Geometry: final body of the model. Coordinates: model frame, mm. A direction names the side the tool comes from. Round coordinates to 2 decimals unless told otherwise and drop trailing zeros. Answer as a JSON object with one key per item and string values.
from build123d import *

# Parameters (mm, degrees)
SKETCH1_R           = 100
BOSS_EXTRUDE1_DEPTH = 50
CUT_EXTRUDE1_DEPTH  = 151
CIRPATTERN1_COUNT   = 6
FILLET1_R           = 3
SKETCH3_R           = 3
CUT_EXTRUDE2_DEPTH  = 151.000000067


with BuildPart() as part:
    # Sketch1 → Boss-Extrude1 (new body)
    with BuildSketch(Plane.XY):
        Circle(SKETCH1_R)
    extrude(amount=BOSS_EXTRUDE1_DEPTH)

    # Sketch2 → Cut-Extrude1 (cut, through all)
    with BuildSketch(Plane.XY.offset(50)):
        with BuildLine():
            Line((0, 90), (0, 10))
            ThreePointArc((0, 10), (2.588190451, 9.659258263), (5, 8.660254038))
            Line((5, 8.660254038), (45, 77.942286341))
            ThreePointArc((45, 77.942286341), (23.293714059, 86.933324366), (0, 90))
        make_face()
    cut_extrude1 = extrude(amount=-CUT_EXTRUDE1_DEPTH, mode=Mode.SUBTRACT)

    # CirPattern1: Cut-Extrude1 ×6 about axis
    cirpattern1_axis = Axis((0, 0, 0), (0, 0, 1))
    for i in range(1, CIRPATTERN1_COUNT):
        add(cut_extrude1.rotate(cirpattern1_axis, i * 360 / CIRPATTERN1_COUNT), mode=Mode.SUBTRACT)

    # Fillet1
    fillet1_edges = [part.edges().sort_by_distance(p)[0] for p in [
        (45, 77.942286341, 25),
        (5, 8.660254038, 25),
        (0, 10, 25),
        (0, 90, 25),
        (-100, 0, 0),
        (90, 0, 25),
        (10, 0, 25),
        (8.660254038, 5, 25),
        (77.942286341, 45, 25),
        (45, -77.942286341, 25),
        (5, -8.660254038, 25),
        (8.660254038, -5, 25),
        (-100, 0, 50),
        (77.942286341, -45, 25),
        (-90, 0, 25),
        (-10, 0, 25),
        (-8.660254038, -5, 25),
        (-77.942286341, -45, 25),
        (-45, -77.942286341, 25),
        (-5, -8.660254038, 25),
        (0, -10, 25),
        (0, -90, 25),
        (-45, 77.942286341, 25),
        (-5, 8.660254038, 25),
        (-8.660254038, 5, 25),
        (-77.942286341, 45, 25),
    ]]
    fillet(fillet1_edges, radius=FILLET1_R)

    # Sketch3 → Cut-Extrude2 (cut, through all)
    with BuildSketch(Plane.XY.offset(50)):
        Circle(SKETCH3_R)
    extrude(amount=-CUT_EXTRUDE2_DEPTH, mode=Mode.SUBTRACT)


solid = part.part
1) Section query A-A (y = -27). Count the separate pieces of the cut face and the enclosed holes in it, and give its area (3 significant figures).
Results:
{"separate pieces": "4", "enclosed holes": "0", "area": "5,330 mm2"}
2) Reachability of faces 4 (the flat face through (24.64, -42.68, 25.35)), 5 (the flat face through (-1, 23, 0)) from +Z, -Z, +X, -X, +Y, -Y: full face, straight path, thin tool, end or side. Return the list, or none.
Results:
{"face 4": "+Z, -Z", "face 5": "-Z, +X, -X, +Y, -Y"}
3) Pull-direction query (Y, two-part tool) for faces 1 (the cylindrical face through (95.38, 30.04, 24.69)), 2 (the cylindrical face through (-63.44, 63.84, 25.35)), 3 (the flat face through (-1, 23, 50)); classes: +Y half, -Y half, draft (parallel to the pull), parting line (faces both ways), or undercut.
Results:
{"face 1": "parting line", "face 2": "undercut", "face 3": "draft"}
4) Ray query, line 1 (Y direction, x = 14, z = 45); line 2 (X direction, y = 23.5, z = 30.5); line 3 (Y direction, x = 11, z = 10). Return the intervals inside material, ascending.
Results:
{"line 1": "-99.02 to -24.25, -8.08 to 0, 8.08 to 24.25, 88.9 to 99.02", "line 2": "-97.2 to -40.7, -13.57 to 0, 13.57 to 40.7, 86.88 to 97.2", "line 3": "-99.39 to -19.05, -6.35 to 0.49, 6.35 to 19.05, 89.33 to 99.39"}
5) Pin query (flat end, axial travel): P1, Ø12, axis at x = 29, z = 33, coming from the +Y side; P2, Ø6, axis at x = 57.5, z = 23.5, coming from the +Y side; P3, Ø15, axis at x = -60.5, z = 33, coming from the -Y side. Return the tip coordinate at first contact, or that it passes through.
Results:
{"P1": "y = 97.32", "P2": "y = 83.84", "P3": "y = -84.8"}
